Study the drawing (mm; zero at the part's minimum x, y, z) and answer. Give positions to 0.01 mm unless a question says otherwise; leave off trailing zeros. Write each loop counter-clockwise with the first axis right and the second up, starting at its lowest first coordinate (ties: lowest second). Pieces come first, ordered by that corner, then holes. Notation, with made-up numbers: (-13, 31.25) -> (6, 31.25) arc R10 ccw to (6, 45.25) -> close; hole circle Ø6 at (22.5, 88.5). An arc over 180 degrees is marked (long way). One line per question, with ' | ' between items.
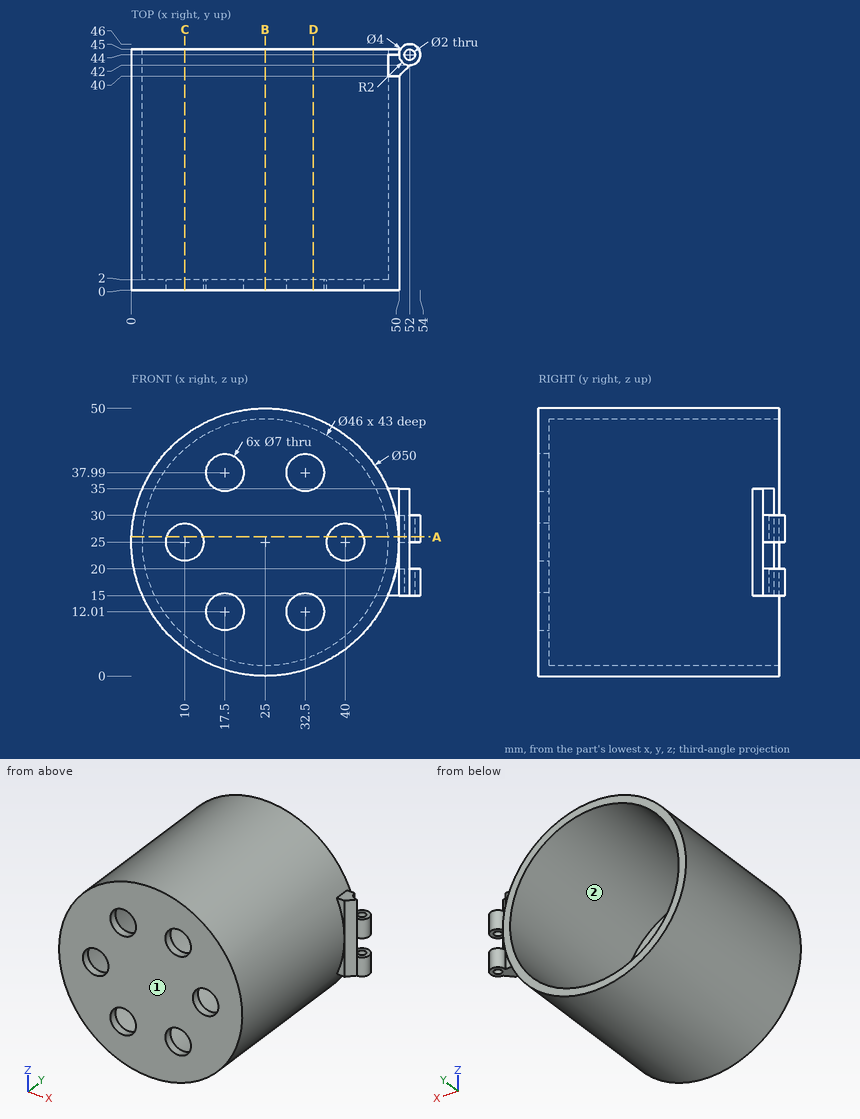
Item 1: Determine the mould class of the marked faces 1 and 2 for opening direction X: pulls with the +X half, pulls with the -X half, needs draft (parallel to the pull), parting line crosses it, or undercut.
Answers below:
face 1: needs draft | face 2: undercut
Item 2: Consider line 1 (X direction, y = 17, z = 25); line 2 (X direction, y = 0.45, z = 25); line 3 (Z direction, x = 32, y = 1) (1 decimal). Determine where each line is inside the solid, lowest interval first. Write a range as [from, to].
Answers below:
line 1: [0, 2], [48, 50] | line 2: [0, 6.5], [13.5, 36.5], [43.5, 50] | line 3: [1, 8.5], [15.5, 34.5], [41.5, 49]
Item 3: Find section B-B (x = 25). Write down the section's boundary in (y, z), then the cut area to 3 significant figures.
Answers below:
outline: (0, 0) -> (45, 0) -> (45, 2) -> (2, 2) -> (2, 48) -> (45, 48) -> (45, 50) -> (0, 50) -> close | area: 272 mm²
Item 4: Find section D-D (x = 34). Write down the section's boundary in (y, z).
Answers below:
outline: (0, 1.68) -> (45, 1.68) -> (45, 3.83) -> (2, 3.83) -> (2, 8.85) -> (0, 8.85) -> close; (0, 15.17) -> (2, 15.17) -> (2, 34.83) -> (0, 34.83) -> close; (0, 41.15) -> (2, 41.15) -> (2, 46.17) -> (45, 46.17) -> (45, 48.32) -> (0, 48.32) -> close
Item 5: Find section C-C (x = 10). Write down the section's boundary in (y, z) (1 decimal).
Answers below:
outline: (0, 5) -> (45, 5) -> (45, 7.6) -> (2, 7.6) -> (2, 21.5) -> (0, 21.5) -> close; (0, 28.5) -> (2, 28.5) -> (2, 42.4) -> (45, 42.4) -> (45, 45) -> (0, 45) -> close
Item 6: Flat-ended cylindrical pins translate along their axes: pin 1 (8 mm diameter, centred on x = 40, z = 25, fed in from +Y); pin 2 (6 mm diameter, centred on x = 41, y = 13.5, fed in from -Z) (1 decimal); pin 3 (0.6 mm diameter, centred on x = 49, z = 21.5, fed in from +Y). Find the tip coordinate at first contact, or state that the pin passes through.
Answers below:
pin 1: y = 2 | pin 2: z = 3.6 | pin 3: y = 45
Item 7: Find section A-A (z = 26). Count the separate pieces of the cut face and the enclosed holes in it.
Answers below:
separate pieces: 3 | enclosed holes: 1
